Work out the finished part from the listing and answer in its coordinate system (mm). Face numbers are marked on the shaded views. A direction names the side the tool comes from. Coordinates: 2 decimals unless noted, no trailing zeros. Loops run counter-clockwise (first coordinate to the right, second up) from the corner with the lowest first, then second, coordinate; pieces in that order, holes last. Notation, with made-up numbers: (17, 52.25) -> (73, 52.25) arc R23 ccw to (73, 85.25) -> close; hole circle Ø9 at (72.5, -29). An arc over 180 degrees is marked (long way). Use a Markdown table: item, result.
from build123d import *

# Parameters (mm, degrees)
SKETCH1_W           = 31
SKETCH1_H           = 43
BOSS_EXTRUDE1_DEPTH = 22
SKETCH2_W           = 27.20800305
SKETCH2_H           = 39
CUT_EXTRUDE1_DEPTH  = 20
SKETCH3_W           = 9.254141904
SKETCH3_H           = 5
CUT_EXTRUDE2_DEPTH  = 20
SKETCH4_W           = 7
SKETCH4_H           = 2
CUT_EXTRUDE3_DEPTH  = 2
SKETCH5_W           = 2
SKETCH5_H           = 2
CUT_EXTRUDE6_DEPTH  = 2
SKETCH6_W           = 5
SKETCH6_H           = 2
SKETCH6_W_2         = 19
CUT_EXTRUDE10_DEPTH = 34
SKETCH10_W          = 1
SKETCH10_H          = 2
CUT_EXTRUDE11_DEPTH = 18
SKETCH11_W          = 1
SKETCH11_H          = 2
CUT_EXTRUDE12_DEPTH = 15
SKETCH12_W          = 1
SKETCH12_H          = 2
BOSS_EXTRUDE3_DEPTH = 2


with BuildPart() as part:
    # Sketch1 → Boss-Extrude1 (new body)
    with BuildSketch(Plane(origin=(0, 0, 0), x_dir=(1, 0, 0), z_dir=(0, 1, 0))):
        Rectangle(SKETCH1_W, SKETCH1_H)
    extrude(amount=BOSS_EXTRUDE1_DEPTH)

    # Sketch2 → Cut-Extrude1 (cut)
    with BuildSketch(Plane(origin=(0, 22, 0), x_dir=(1, 0, 0), z_dir=(0, 1, 0))):
        Rectangle(SKETCH2_W, SKETCH2_H)
    extrude(amount=-CUT_EXTRUDE1_DEPTH, mode=Mode.SUBTRACT)

    # Sketch3 → Cut-Extrude2 (cut)
    with BuildSketch(Plane.XY.offset(21.5)):
        with Locations((0.126254012, 7.5)):
            Rectangle(SKETCH3_W, SKETCH3_H)
    extrude(amount=-CUT_EXTRUDE2_DEPTH, mode=Mode.SUBTRACT)

    # Sketch4 → Cut-Extrude3 (cut)
    with BuildSketch(Plane.XY.offset(21.5)):
        with Locations((-12, 21)):
            Rectangle(SKETCH4_W, SKETCH4_H)
        with Locations((0, 21)):
            Rectangle(SKETCH4_W, SKETCH4_H)
        with Locations((12, 21)):
            Rectangle(SKETCH4_W, SKETCH4_H)
    extrude(amount=-CUT_EXTRUDE3_DEPTH, mode=Mode.SUBTRACT)

    # Sketch5 → Cut-Extrude6 (cut)
    with BuildSketch(Plane(origin=(0, 0, -21.5), x_dir=(-1, 0, 0), z_dir=(0, 0, -1))):
        with Locations((14.5, 21)):
            Rectangle(SKETCH5_W, SKETCH5_H)
        Polygon((-8.5, 22), (-8.5, 20), (-6.500281768, 20), (6.499718232, 20), (8.5, 20), (8.5, 22), align=None)
        with Locations((-14.5, 21)):
            Rectangle(SKETCH5_W, SKETCH5_H)
        Polygon((6.499718232, 20), (-6.500281768, 20), (-6.500281768, 19.64343591), (-6.500281768, 18), (6.499718232, 18), align=None)
    extrude(amount=-CUT_EXTRUDE6_DEPTH, mode=Mode.SUBTRACT)

    # Sketch6 → Cut-Extrude10 (cut)
    with BuildSketch(Plane.ZY.offset(15.5)):
        with Locations((-17, 21)):
            Rectangle(SKETCH6_W, SKETCH6_H)
        with Locations((0, 21)):
            Rectangle(SKETCH6_W_2, SKETCH6_H)
        with Locations((12, 21)):
            Rectangle(SKETCH6_W, SKETCH6_H)
    extrude(amount=-CUT_EXTRUDE10_DEPTH, mode=Mode.SUBTRACT)

    # Sketch10 → Cut-Extrude11 (cut)
    with BuildSketch(Plane(origin=(0, 2, 0), x_dir=(1, 0, 0), z_dir=(0, 1, 0))):
        with Locations((14.104001525, -12.5)):
            Rectangle(SKETCH10_W, SKETCH10_H)
    extrude(amount=CUT_EXTRUDE11_DEPTH, mode=Mode.SUBTRACT)

    # Sketch11 → Cut-Extrude12 (cut)
    with BuildSketch(Plane(origin=(0, 20, 0), x_dir=(1, 0, 0), z_dir=(0, 1, 0))):
        with Locations((-14.104001525, -12.5)):
            Rectangle(SKETCH11_W, SKETCH11_H)
    extrude(amount=-CUT_EXTRUDE12_DEPTH, mode=Mode.SUBTRACT)

    # Sketch12 → Boss-Extrude3 (add)
    with BuildSketch(Plane(origin=(0, 2, 0), x_dir=(1, 0, 0), z_dir=(0, 1, 0))):
        with Locations((14.104001525, -12.5)):
            Rectangle(SKETCH12_W, SKETCH12_H)
    extrude(amount=BOSS_EXTRUDE3_DEPTH)


solid = part.part
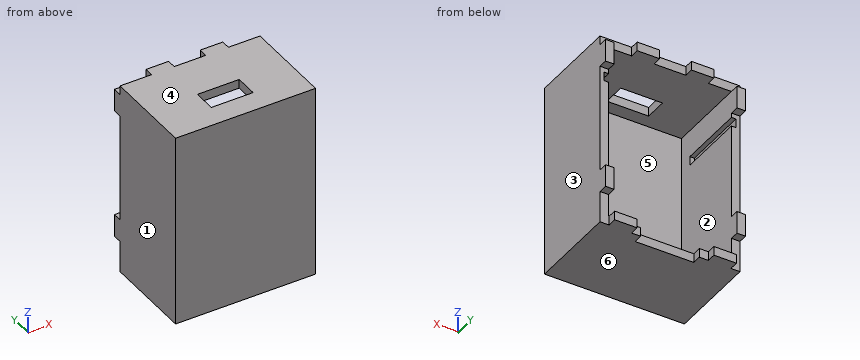
Q1. Section B-B on y = 11.5 is taken. Determine the outline of the cut face in (x, z).
Solved:
| item | result |
|---|---|
| outline | (-15.5, -21.5) -> (15.5, -21.5) -> (15.5, 21.5) -> (-15.5, 21.5) -> close; hole (-14.6, 11.5) -> (-13.6, 11.5) -> (-13.6, -19.5) -> (13.6, -19.5) -> (13.6, 11.5) -> (14.6, 11.5) -> (14.6, 13.5) -> (13.6, 13.5) -> (13.6, 19.5) -> (-13.6, 19.5) -> (-13.6, 13.5) -> (-14.6, 13.5) -> close |
Q2. Consider line 1 (X direction, y = 18.25, z = -15); line 2 (Z direction, x = 6, y = 10.5); line 3 (Y direction, x = -4, z = 0.5). Determine where each line is inside the solid, lowest interval first. Write a range as [from, to].
Solved:
| item | result |
|---|---|
| line 1 | [-15.5, -13.6], [13.6, 15.5] |
| line 2 | [-21.5, -19.5], [19.5, 21.5] |
| line 3 | [0, 2] |
Q3. Section C-C on z = 15 is taken. Determine the outline of the cut face in (x, y).
Solved:
| item | result |
|---|---|
| outline | (-15.5, 0) -> (15.5, 0) -> (15.5, 22) -> (13.6, 22) -> (13.6, 2) -> (-13.6, 2) -> (-13.6, 22) -> (-15.5, 22) -> close |
Q4. Determine the mould class of the marked faces 3, 4, 5 and 6 for opening direction Z: pulls with the +Z half, pulls with the -Z half, needs draft (parallel to the pull), parting line crosses it, or undercut.
Solved:
| item | result |
|---|---|
| face 3 | needs draft |
| face 4 | pulls with the +Z half |
| face 5 | undercut |
| face 6 | pulls with the -Z half |
Q5. Given pin 1 Ø2 at (x, y) = (15, 21.5) entering from -Z; pin 2 Ø5 at (x, z) = (9.5, -2) entering from +Y; pin 3 Ø1.5 at (x, y) = (-14, 20.5) entering from -Z; pin 4 Ø0.6 at (x, y) = (14.5, 21) entering from +Z, each flat-ended and moving along its own axis, determine where each tip first touches the part or whether it passes through.
Solved:
| item | result |
|---|---|
| pin 1 | z = -14.5 |
| pin 2 | y = 2 |
| pin 3 | z = -21.5 |
| pin 4 | z = 19.5 |
Q6. Section D-D on x = -12.5 is taken. Determine the outline of the cut face in (y, z).
Solved:
| item | result |
|---|---|
| outline | (0, -21.5) -> (22, -21.5) -> (22, -19.5) -> (2, -19.5) -> (2, 19.5) -> (20, 19.5) -> (20, 21.5) -> (0, 21.5) -> close |
Q7. Section A-A on x = -4 is taken. Determine the outline of the cut face in (y, z).
Solved:
| item | result |
|---|---|
| outline | (0, -21.5) -> (18, -21.5) -> (18, -19.5) -> (2, -19.5) -> (2, 19.5) -> (5, 19.5) -> (5, 21.5) -> (0, 21.5) -> close; (10, 19.5) -> (22, 19.5) -> (22, 21.5) -> (10, 21.5) -> close |
Q8. For the marked faces 1 and 2, determine the directions among +Z, -Z, +X, -X, +Y, -Y from which every point of the face is accessible in a straight line to the end or side of a thin tool.
Solved:
| item | result |
|---|---|
| face 1 | +Z, -Z, -X, +Y, -Y |
| face 2 | +Y |
